Read the model definition and answer for the solid it produces. Units are mm, in the model's axes. Give positions to 0.01 mm unless a question says otherwise; leave off trailing zeros. Write each loop counter-clockwise with the first axis right and the second up, starting at its lowest first coordinate (ties: lowest second). Pieces come first, ordered by that corner, then holes. Notation, with made-up numbers: (14.25, 38.25) - (24.25, 38.25) arc R29 cw to (24.25, 59.25) - close; hole circle Ø9 at (5, -19). An arc over 180 degrees is marked (long way). Use CSV: the item, a comma, the result in double quotes. Start each with the question number.
from build123d import *

# Parameters (mm, degrees)
SKETCH1_W           = 30
SKETCH1_H           = 6
BOSS_EXTRUDE1_DEPTH = 7.76
SKETCH2_R           = 2.65
CUT_EXTRUDE1_DEPTH  = 8
SKETCH3_W           = 7.76
SKETCH3_H           = 6
BOSS_EXTRUDE2_DEPTH = 6
SKETCH4_W           = 7.76
SKETCH4_H           = 6
BOSS_EXTRUDE3_DEPTH = 6
SKETCH5_R           = 2.65
CUT_EXTRUDE2_DEPTH  = 8
SKETCH6_W           = 42
SKETCH6_H           = 7.76
BOSS_EXTRUDE4_DEPTH = 0.5
SKETCH7_W           = 7.76
SKETCH7_H           = 6.5
BOSS_EXTRUDE5_DEPTH = 0.5
SKETCH8_W           = 42.5
SKETCH8_H           = 7.76
BOSS_EXTRUDE6_DEPTH = 0.5
SKETCH9_W           = 7.76
SKETCH9_H           = 7
BOSS_EXTRUDE7_DEPTH = 0.5
FILLET1_R           = 3


with BuildPart() as part:
    # Sketch1 → Boss-Extrude1 (new body)
    with BuildSketch(Plane.XY):
        Rectangle(SKETCH1_W, SKETCH1_H)
    extrude(amount=BOSS_EXTRUDE1_DEPTH)

    # Sketch2 → Cut-Extrude1 (cut)
    with BuildSketch(Plane.XY.offset(7.76)):
        Circle(SKETCH2_R)
        with Locations((7.97, 0)):
            Circle(SKETCH2_R)
        with Locations((-7.97, 0)):
            Circle(SKETCH2_R)
    extrude(amount=-CUT_EXTRUDE1_DEPTH, mode=Mode.SUBTRACT)

    # Sketch3 → Boss-Extrude2 (add)
    with BuildSketch(Plane.ZY.offset(15)):
        with Locations((3.88, 0)):
            Rectangle(SKETCH3_W, SKETCH3_H)
    extrude(amount=BOSS_EXTRUDE2_DEPTH)

    # Sketch4 → Boss-Extrude3 (add)
    with BuildSketch(Plane(origin=(15, 0, 0), x_dir=(0, 0, -1), z_dir=(1, 0, 0))):
        with Locations((-3.88, 0)):
            Rectangle(SKETCH4_W, SKETCH4_H)
    extrude(amount=BOSS_EXTRUDE3_DEPTH)

    # Sketch5 → Cut-Extrude2 (cut)
    with BuildSketch(Plane.XY.offset(7.76)):
        with Locations((-15.94, 0)):
            Circle(SKETCH5_R)
        with Locations((15.94, 0)):
            Circle(SKETCH5_R)
    extrude(amount=-CUT_EXTRUDE2_DEPTH, mode=Mode.SUBTRACT)

    # Sketch6 → Boss-Extrude4 (add)
    with BuildSketch(Plane(origin=(0, 3, 0), x_dir=(1, 0, 0), z_dir=(0, 1, 0))):
        with Locations((0, -3.88)):
            Rectangle(SKETCH6_W, SKETCH6_H)
    extrude(amount=BOSS_EXTRUDE4_DEPTH)

    # Sketch7 → Boss-Extrude5 (add)
    with BuildSketch(Plane(origin=(21, 0, 0), x_dir=(0, 0, -1), z_dir=(1, 0, 0))):
        with Locations((-3.88, 0.25)):
            Rectangle(SKETCH7_W, SKETCH7_H)
    extrude(amount=BOSS_EXTRUDE5_DEPTH)

    # Sketch8 → Boss-Extrude6 (add)
    with BuildSketch(Plane.XZ.offset(3)):
        with Locations((0.25, 3.88)):
            Rectangle(SKETCH8_W, SKETCH8_H)
    extrude(amount=BOSS_EXTRUDE6_DEPTH)

    # Sketch9 → Boss-Extrude7 (add)
    with BuildSketch(Plane.ZY.offset(21)):
        with Locations((3.88, 0)):
            Rectangle(SKETCH9_W, SKETCH9_H)
    extrude(amount=BOSS_EXTRUDE7_DEPTH)

    # Fillet1
    fillet1_edges = [part.edges().sort_by_distance(p)[0] for p in [
        (-21.5, 3.5, 3.88),
        (21.5, 3.5, 3.88),
    ]]
    fillet(fillet1_edges, radius=FILLET1_R)


solid = part.part
(1) Consider probe 1 along Y at (x, z) = (-16, 5.25); probe 2 along X at (y, z) = (2, 0.75); probe 3 along X at (y, z) = (-2, 6.5). Determine where each line is inside the solid, lowest interval first.
(2) For a pull along Y with two mould halves and no side action, classify faces 1 (the face through (0, -3, 7.76)), 2 (the face through (2.45, -1.01, 3.93)), 3 (the face through (20.64, 2.6, 3.83)), 4 (the face through (0, -3.5, 4)) as pulls with the +Y half, pulls with the -Y half, needs draft (parallel to the pull), parting line crosses it, or undercut.
(3) The part is cut by section C-C on z = 4.25. Write down the section's boundary in (x, y), plus the area to 3 significant figures.
(4) The part is cut by section B-B on x = -7.97. Write down the section's boundary in (y, z).
(5) The part is cut by section A-A on y = 0. Write down the section's boundary in (x, z).
(6) Given P1, Ø1, axis at x = -13.5, y = 2, coming from the -Z side; P2, Ø1.5, axis at y = 2, z = 5.5, coming from the +X side, each flat-ended and moving along its own axis, determine where each tip first touches the part or whether it passes through.
(7) The part is cut by section D-D on y = 2. Write down the section's boundary in (x, z), plus the area to 3 significant figures.
Reported:
1,probe 1,"-3.5 to -2.65, 2.65 to 3.5"
1,probe 2,"-21.1 to -17.68, -14.2 to -9.71, -6.23 to -1.74, 1.74 to 6.23, 9.71 to 14.2, 17.68 to 21.1"
1,probe 3,"-21.5 to -17.68, -14.2 to -9.71, -6.23 to -1.74, 1.74 to 6.23, 9.71 to 14.2, 17.68 to 21.5"
2,face 1,"needs draft"
2,face 2,"undercut"
2,face 3,"pulls with the +Y half"
2,face 4,"pulls with the -Y half"
3,outline,"(-21.5, -3.5) - (21.5, -3.5) - (21.5, 0.5) arc R3 ccw to (18.5, 3.5) - (-18.5, 3.5) arc R3 ccw to (-21.5, 0.5) - close; hole circle Ø5.3 at (-15.94, 0); hole circle Ø5.3 at (-7.97, 0); hole circle Ø5.3 at (0, 0); hole circle Ø5.3 at (7.97, 0); hole circle Ø5.3 at (15.94, 0)"
3,area,"187 mm²"
4,outline,"(-3.5, 0) - (-2.65, 0) - (-2.65, 7.76) - (-3.5, 7.76) - close; (2.65, 0) - (3.5, 0) - (3.5, 7.76) - (2.65, 7.76) - close"
5,outline,"(-21.5, 0) - (-18.59, 0) - (-18.59, 7.76) - (-21.5, 7.76) - close; (-13.29, 0) - (-10.62, 0) - (-10.62, 7.76) - (-13.29, 7.76) - close; (-5.32, 0) - (-2.65, 0) - (-2.65, 7.76) - (-5.32, 7.76) - close; (2.65, 0) - (5.32, 0) - (5.32, 7.76) - (2.65, 7.76) - close; (10.62, 0) - (13.29, 0) - (13.29, 7.76) - (10.62, 7.76) - close; (18.59, 0) - (21.5, 0) - (21.5, 7.76) - (18.59, 7.76) - close"
6,P1,"z = 0"
6,P2,"x = 21.4"
7,outline,"(-21.1, 0) - (-17.68, 0) - (-17.68, 7.76) - (-21.1, 7.76) - close; (-14.2, 0) - (-9.71, 0) - (-9.71, 7.76) - (-14.2, 7.76) - close; (-6.23, 0) - (-1.74, 0) - (-1.74, 7.76) - (-6.23, 7.76) - close; (1.74, 0) - (6.23, 0) - (6.23, 7.76) - (1.74, 7.76) - close; (9.71, 0) - (14.2, 0) - (14.2, 7.76) - (9.71, 7.76) - close; (17.68, 0) - (21.1, 0) - (21.1, 7.76) - (17.68, 7.76) - close"
7,area,"193 mm²"
